Part model, mm, in its own coordinate system. Face numbers are marked on the shaded views. A direction names the side the tool comes from. Give positions to 0.01 mm unless a question says otherwise; leave off trailing zeros. Write each loop counter-clockwise with the first axis right and the second up, starting at its lowest first coordinate (ties: lowest second). Pieces come first, ordered by that corner, then holes. Notation, with made-up numbers: M -23,0.25 L -12,0.25 A23 ccw -12,33.25 Z; hole C 73.5,-27.75 d9. An arc over 180 degrees is marked long. Use CSV: the item, a comma, the result in double quotes. Start each with the question number.
1. Band-saw the part on A-A, the plane y = -18. List the corners of the cut face in (x, z), then the cut area to 3 significant figures.
2. Band-saw the part on C-C, the plane x = 16. List the corners of the cut face in (y, z).
3. Mould opens along X. For the marked faces 4, 5 and 6 say: pulls with the +X half, pulls with the -X half, needs draft (parallel to the pull), parting line crosses it, or undercut.
4. 3-axis set-ups, long thin cutter, end or side, ignore diameter. For the marked faces 1, 2 and 3: which of +Z, -Z, +X, -X, +Y, -Y reach the whole face in a straight line?
5. Drop flat-ended pins along their axis: pin 1 Ø2 at (x, z) = (40.5, 4.5) entering from -Y; pin 2 Ø2.5 at (x, z) = (10, 3.5) entering from -Y; pin 3 Ø4 at (y, z) = (-23.5, 5.5) entering from +X. Give the stop position or say it passes through.
6. Band-saw the part on B-B, the plane z = 3. List the corners of the cut face in (x, y).
7. Band-saw the part on D-D, the plane y = -1.5. List the corners of the cut face in (x, z).
8. Drill centre lines: line 1 along X through (y, z) = (-1, 6.75); line 2 along X through (y, z) = (-7.5, 4.5); line 3 along X through (y, z) = (-13, 2.25). Where is each one in solid material? Low to high. Write a range as from..to.
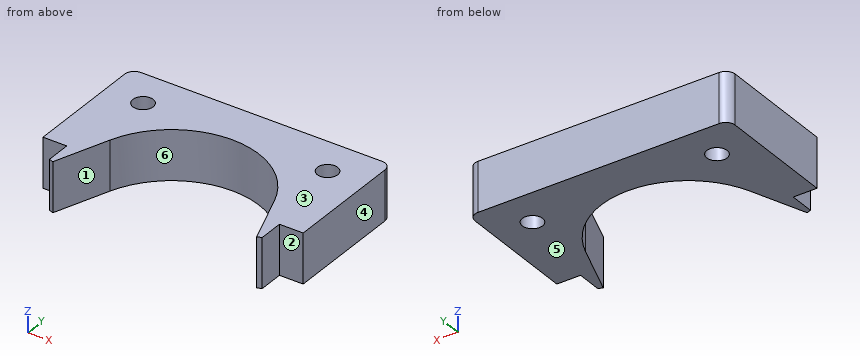
from build123d import *

# Parameters (mm, degrees)
SKETCH1_R           = 2.15
BOSS_EXTRUDE1_DEPTH = 10.5
FILLET1_R           = 2


with BuildPart() as part:
    # Sketch1 → Boss-Extrude1 (new body)
    with BuildSketch(Plane.XY):
        with BuildLine():
            Line((13.944137731, -26.361003887), (14.869335388, -26.697748295))
            Line((14.869335388, -26.697748295), (19.041515783, -15.234776871))
            ThreePointArc((19.041515783, -15.234776871), (36.418598187, -3.067212779), (53.795680592, -15.234776871))
            Line((53.795680592, -15.234776871), (57.967860986, -26.697748295))
            Line((57.967860986, -26.697748295), (58.893058643, -26.361003887))
            Line((58.893058643, -26.361003887), (58.893058643, -21.090651307))
            Line((58.893058643, -21.090651307), (63.918598187, -21.090651307))
            Line((63.918598187, -21.090651307), (63.918598187, 5.940482376))
            Line((63.918598187, 5.940482376), (8.918598187, 5.940482376))
            Line((8.918598187, 5.940482376), (8.918598187, -21.090651307))
            Line((8.918598187, -21.090651307), (13.944137731, -21.090651307))
            Line((13.944137731, -21.090651307), (13.944137731, -26.361003887))
        make_face()
        with Locations((55.918598187, -2.059517624)):
            Circle(SKETCH1_R, mode=Mode.SUBTRACT)
        with Locations((16.918598187, -2.059517624)):
            Circle(SKETCH1_R, mode=Mode.SUBTRACT)
    extrude(amount=BOSS_EXTRUDE1_DEPTH)

    # Fillet1
    fillet1_edges = [part.edges().sort_by_distance(p)[0] for p in [
        (8.918598187, 5.940482376, 5.25),
        (63.918598187, 5.940482376, 5.25),
    ]]
    fillet(fillet1_edges, radius=FILLET1_R)


solid = part.part
Output:
1,outline,"M 8.92,0 L 18.04,0 L 18.04,10.5 L 8.92,10.5 Z; M 54.8,0 L 63.92,0 L 63.92,10.5 L 54.8,10.5 Z"
1,area,"191 mm²"
2,outline,"M -23.59,0 L -4,0 L -4,10.5 L -23.59,10.5 Z; M -0.12,0 L 5.94,0 L 5.94,10.5 L -0.12,10.5 Z"
3,face 4,"pulls with the +X half"
3,face 5,"needs draft"
3,face 6,"undercut"
4,face 1,"+Z, -Z, -Y"
4,face 2,"+Z, -Z, +X, -Y"
4,face 3,"+Z, +X, -X, +Y, -Y"
5,pin 1,"stops at y = -3.78"
5,pin 2,"stops at y = -21.09"
5,pin 3,"stops at x = 58.89"
6,outline,"M 8.92,-21.09 L 13.94,-21.09 L 13.94,-26.36 L 14.87,-26.7 L 19.04,-15.23 A18.49 cw 53.8,-15.23 L 57.97,-26.7 L 58.89,-26.36 L 58.89,-21.09 L 63.92,-21.09 L 63.92,3.94 A2 ccw 61.92,5.94 L 10.92,5.94 A2 ccw 8.92,3.94 Z; hole C 16.92,-2.06 d4.3; hole C 55.92,-2.06 d4.3"
7,outline,"M 8.92,0 L 14.84,0 L 14.84,10.5 L 8.92,10.5 Z; M 18.99,0 L 53.84,0 L 53.84,10.5 L 18.99,10.5 Z; M 57.99,0 L 63.92,0 L 63.92,10.5 L 57.99,10.5 Z"
8,line 1,"x = 8.92..15.05, 18.79..54.05, 57.79..63.92"
8,line 2,"x = 8.92..24.41, 48.43..63.92"
8,line 3,"x = 8.92..20.03, 52.81..63.92"
